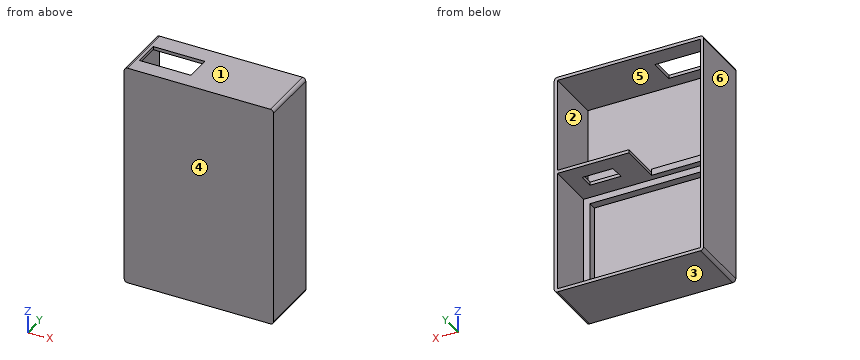
from build123d import *

# Parameters (mm, degrees)
SKETCH1_W           = 46.2
SKETCH1_H           = 39.2
SKETCH1_W_2         = 40.2
SKETCH1_H_2         = 33.2
BOSS_EXTRUDE1_DEPTH = 2.5
SKETCH3_W           = 46.2
SKETCH3_H           = 39.2
BOSS_EXTRUDE2_DEPTH = 1
SKETCH4_W           = 46.2
SKETCH4_H           = 39.2
SKETCH4_W_2         = 44.2
SKETCH4_H_2         = 37.2
BOSS_EXTRUDE3_DEPTH = 15
SKETCH5_W           = 9.5
SKETCH5_H           = 4.5
CUT_EXTRUDE1_DEPTH  = 15
SKETCH6_W           = 46.2
SKETCH6_H           = 30
BOSS_EXTRUDE4_DEPTH = 1
SKETCH7_W           = 46.2
SKETCH7_H           = 30
SKETCH7_W_2         = 44.2
SKETCH7_H_2         = 28
BOSS_EXTRUDE5_DEPTH = 17.5
SKETCH8_W           = 22.1
SKETCH8_H           = 2
CUT_EXTRUDE2_DEPTH  = 13
SKETCH9_W           = 22.1
SKETCH9_H           = 1
CUT_EXTRUDE3_DEPTH  = 17.5
SKETCH10_W          = 16
SKETCH10_H          = 8
CUT_EXTRUDE4_DEPTH  = 10
FILLET1_R           = 1


with BuildPart() as part:
    # Sketch1 → Boss-Extrude1 (new body)
    with BuildSketch(Plane(origin=(0, 0, 0), x_dir=(1, 0, 0), z_dir=(0, 1, 0))):
        Rectangle(SKETCH1_W, SKETCH1_H)
        Rectangle(SKETCH1_W_2, SKETCH1_H_2, mode=Mode.SUBTRACT)
    extrude(amount=BOSS_EXTRUDE1_DEPTH)

    # Sketch3 → Boss-Extrude2 (add)
    with BuildSketch(Plane.XZ):
        Rectangle(SKETCH3_W, SKETCH3_H)
    extrude(amount=BOSS_EXTRUDE2_DEPTH)

    # Sketch4 → Boss-Extrude3 (add)
    with BuildSketch(Plane(origin=(0, 2.5, 0), x_dir=(1, 0, 0), z_dir=(0, 1, 0))):
        Rectangle(SKETCH4_W, SKETCH4_H)
        Rectangle(SKETCH4_W_2, SKETCH4_H_2, mode=Mode.SUBTRACT)
    extrude(amount=BOSS_EXTRUDE3_DEPTH)

    # Sketch5 → Cut-Extrude1 (cut)
    with BuildSketch(Plane(origin=(0, 0, 18.6), x_dir=(-1, 0, 0), z_dir=(0, 0, -1))):
        with Locations((-12.35, 10.25)):
            Rectangle(SKETCH5_W, SKETCH5_H)
    extrude(amount=-CUT_EXTRUDE1_DEPTH, mode=Mode.SUBTRACT)

    # Sketch6 → Boss-Extrude4 (add)
    with BuildSketch(Plane.XZ.offset(1)):
        with Locations((0, 34.6)):
            Rectangle(SKETCH6_W, SKETCH6_H)
    extrude(amount=-BOSS_EXTRUDE4_DEPTH)

    # Sketch7 → Boss-Extrude5 (add)
    with BuildSketch(Plane(origin=(0, 0, 0), x_dir=(1, 0, 0), z_dir=(0, 1, 0))):
        with Locations((0, -34.6)):
            Rectangle(SKETCH7_W, SKETCH7_H)
        with Locations((0, -34.6)):
            Rectangle(SKETCH7_W_2, SKETCH7_H_2, mode=Mode.SUBTRACT)
    extrude(amount=BOSS_EXTRUDE5_DEPTH)

    # Sketch8 → Cut-Extrude2 (cut)
    with BuildSketch(Plane(origin=(0, 17.5, 0), x_dir=(1, 0, 0), z_dir=(0, 1, 0))):
        with Locations((-11.05, -19.6)):
            Rectangle(SKETCH8_W, SKETCH8_H)
    extrude(amount=-CUT_EXTRUDE2_DEPTH, mode=Mode.SUBTRACT)

    # Sketch9 → Cut-Extrude3 (cut)
    with BuildSketch(Plane(origin=(0, 17.5, 0), x_dir=(1, 0, 0), z_dir=(0, 1, 0))):
        with Locations((11.05, -20.1)):
            Rectangle(SKETCH9_W, SKETCH9_H)
    extrude(amount=-CUT_EXTRUDE3_DEPTH, mode=Mode.SUBTRACT)

    # Sketch10 → Cut-Extrude4 (cut)
    with BuildSketch(Plane.XY.offset(49.6)):
        with Locations((-13.1, 8)):
            Rectangle(SKETCH10_W, SKETCH10_H)
    extrude(amount=-CUT_EXTRUDE4_DEPTH, mode=Mode.SUBTRACT)

    # Fillet1
    fillet1_edges = [part.edges().sort_by_distance(p)[0] for p in [
        (-23.1, 8.25, -19.6),
        (23.1, 8.25, -19.6),
        (-23.1, 8.25, 49.6),
        (23.1, 8.25, 49.6),
    ]]
    fillet(fillet1_edges, radius=FILLET1_R)


solid = part.part
The model under review builds one solid part; all positions refer to its coordinate system, in mm. Face numbers are marked on the shaded views. A direction names the side the tool comes from. Round coordinates to 2 decimals unless told otherwise and drop trailing zeros. Write each loop counter-clockwise with the first axis right and the second up, starting at its lowest first coordinate (ties: lowest second). Pieces come first, ordered by that corner, then holes. Notation, with made-up numbers: (-8.5, 77.5) - (49.5, 77.5) arc R7 cw to (49.5, 82.5) - close; hole circle Ø3 at (-10, -7.75). An arc over 180 degrees is marked (long way). One line per item, written item: value. Start each with the question number.
1. Consider section C-C on z = -4. Write out the cut boundary in (x, y).
2. Machinability: for the marked faces 5 and 6, which of the approach directions +Z, -Z, +X, -X, +Y, -Y give a long, thin tool a straight path to every point of the face, cutting with its end or side? Answer none if there is none.
3. Consider section B-B on y = 3.25. Write out the cut boundary in (x, z), and give its area (3 significant figures).
4. The part is to be moulded in two halves that separate along Z. For the marked faces 1, 2, 3 and 4, say which applies: released by +Z, released by -Z, zero draft, split by the parting line, or undercut.
5. To check wall thickness, follow L1, parallel to Z at x = 10, y = 13.5; L2, parallel to Z at x = -4, y = 12.75; L3, parallel to Z at x = -2.5, y = 3.25. State the ranges of each line that lie inside material, in increasing order. Write a range as from..to.
6. Consider section D-D on y = 11. Write out the cut boundary in (x, z), and give its area (3 significant figures).
7. Consider section A-A on x = 14. Write out the cut boundary in (y, z), and give its area (3 significant figures).
8. Clearance check with flat-ended pins moving along their axes: P1, Ø6, axis at x = -7.5, z = 33.5, coming from the +Y side; P2, Ø0.6, axis at x = -8, z = 20, coming from the +Y side. State where each tip first meets the part, or that it passes through.
Checks:
1. outline: (-23.1, -1) - (23.1, -1) - (23.1, 17.5) - (22.1, 17.5) - (22.1, 2.5) - (20.1, 2.5) - (20.1, 0) - (-20.1, 0) - (-20.1, 2.5) - (-22.1, 2.5) - (-22.1, 17.5) - (-23.1, 17.5) - close
2. face 5: +Y
2. face 6: +Z, -Z, -X, +Y, -Y
3. outline: (-23.1, -18.6) arc R1 ccw to (-22.1, -19.6) - (22.1, -19.6) arc R1 ccw to (23.1, -18.6) - (23.1, 48.6) arc R1 ccw to (22.1, 49.6) - (-22.1, 49.6) arc R1 ccw to (-23.1, 48.6) - close; hole (-22.1, -18.6) - (22.1, -18.6) - (22.1, 18.6) - (-22.1, 18.6) - close; hole (-22.1, 20.6) - (0, 20.6) - (0, 19.6) - (22.1, 19.6) - (22.1, 48.6) - (-22.1, 48.6) - close
3. area: 292 mm^2
4. face 1: released by +Z
4. face 2: undercut
4. face 3: released by -Z
4. face 4: zero draft
5. L1: z = -19.6..-18.6, 18.6..19.6, 48.6..49.6
5. L2: z = -19.6..-18.6, 48.6..49.6
5. L3: z = -19.6..-18.6, 18.6..20.6, 48.6..49.6
6. outline: (-23.1, -18.6) arc R1 ccw to (-22.1, -19.6) - (22.1, -19.6) arc R1 ccw to (23.1, -18.6) - (23.1, 48.6) arc R1 ccw to (22.1, 49.6) - (-5.1, 49.6) - (-5.1, 48.6) - (22.1, 48.6) - (22.1, 19.6) - (17.1, 19.6) - (17.1, 18.6) - (22.1, 18.6) - (22.1, -18.6) - (-22.1, -18.6) - (-22.1, 48.6) - (-21.1, 48.6) - (-21.1, 49.6) - (-22.1, 49.6) arc R1 ccw to (-23.1, 48.6) - close; (0, 18.6) - (7.6, 18.6) - (7.6, 19.6) - (0, 19.6) - close
6. area: 223 mm^2
7. outline: (-1, -19.6) - (17.5, -19.6) - (17.5, -18.6) - (2.5, -18.6) - (2.5, -16.6) - (0, -16.6) - (0, 16.6) - (2.5, 16.6) - (2.5, 18.6) - (8, 18.6) - (8, 19.6) - (0, 19.6) - (0, 48.6) - (17.5, 48.6) - (17.5, 49.6) - (-1, 49.6) - close; (12.5, 18.6) - (17.5, 18.6) - (17.5, 19.6) - (12.5, 19.6) - close
7. area: 127 mm^2
8. P1: stops at y = 0
8. P2: stops at y = 4.5
